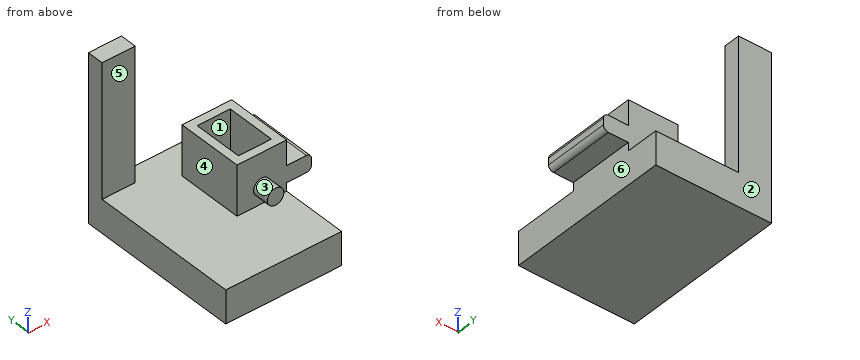
from build123d import *

# Parameters (mm, degrees)
F0_W      = 70
F0_H      = 100
F1_DEPTH  = 20
F2_W      = 20
F2_H      = 10
F3_DEPTH  = 80
F4_W      = 30
F4_H      = 40
F5_DEPTH  = 30
F6_W      = 20
F6_H      = 30
F7_DEPTH  = 30
F8_W      = 40
F8_H      = 10
F9_DEPTH  = 15
F10_R     = 5
F11_DEPTH = 10
F12_R     = 3


with BuildPart() as f1:
    # F0 (on Top) → F1 (new body)
    with BuildSketch(Plane.XY):
        with Locations((35, 50)):
            Rectangle(F0_W, F0_H)
    extrude(amount=F1_DEPTH)

    # F2 (on face) → F3 (join)
    with BuildSketch(Plane.XY.offset(20)):
        with Locations((10, 95)):
            Rectangle(F2_W, F2_H)
    extrude(amount=F3_DEPTH)

    # F4 (on face) → F5 (join)
    with BuildSketch(Plane.XY.offset(20)):
        with Locations((55, 60)):
            Rectangle(F4_W, F4_H)
    extrude(amount=F5_DEPTH)

    # F6 (on face) → F7 (cut)
    with BuildSketch(Plane.XY.offset(50)):
        with Locations((55, 60)):
            Rectangle(F6_W, F6_H)
    extrude(amount=-F7_DEPTH, mode=Mode.SUBTRACT)

    # F8 (on face) → F9 (join)
    with BuildSketch(Plane.YZ.offset(70)):
        with Locations((60, 30)):
            Rectangle(F8_W, F8_H)
    extrude(amount=F9_DEPTH)

    # F10 (on face) → F11 (join)
    with BuildSketch(Plane.XZ.offset(-40)):
        with Locations((55, 30)):
            Circle(F10_R)
    extrude(amount=F11_DEPTH)

    # F12
    f12_edges = [f1.edges().sort_by_distance(p)[0] for p in [
        (85, 60, 35),
        (85, 60, 25),
    ]]
    fillet(f12_edges, radius=F12_R)


solid = f1.part
The listing builds one solid part. Answer for the finished solid, in the listing's coordinates (mm). Face numbers are marked on the shaded views. A direction names the side the tool comes from. Give positions to 0.01 mm unless a question says otherwise; leave off trailing zeros. Loops run counter-clockwise (first coordinate to the right, second up) from the corner with the lowest first, then second, coordinate; pieces in that order, holes last. Notation, with made-up numbers: M 74,-19 L 92,-19 A15 cw 92,3 Z; hole C 0.25,60 d1. An arc over 180 degrees is marked long. Answer as CSV lines item,"result".
Item 1: Given pin 1 Ø10 at (x, y) = (55.5, 61) entering from +Z; pin 2 Ø16 at (x, z) = (54.5, 41.5) entering from +Y; pin 3 Ø10 at (x, y) = (35.5, 32) entering from -Z; pin 4 Ø24 at (x, y) = (62.5, 62) entering from +Z, each flat-ended and moving along its own axis, determine where each tip first touches the part or whether it passes through.
Values follow:
pin 1,"stops at z = 20"
pin 2,"stops at y = 80"
pin 3,"stops at z = 0"
pin 4,"stops at z = 50"
Item 2: Straight lines are drawn through the part: line 1 along Y through (x, z) = (60, 23); line 2 along Y through (x, z) = (59, 32); line 3 along Z through (x, y) = (71.5, 70). For each, find the intervals that lie inside material, in ascending order. Write a range as [from, to].
Values follow:
line 1,"y = [40, 45], [75, 80]"
line 2,"y = [30, 45], [75, 80]"
line 3,"z = [25, 35]"
Item 3: The part is cut by section C-C (y = 61). Give the vertices of the cut face in (x, z), and give its area (3 significant figures).
Values follow:
outline,"M 0,0 L 70,0 L 70,25 L 82,25 A3 ccw 85,28 L 85,32 A3 ccw 82,35 L 70,35 L 70,50 L 65,50 L 65,20 L 45,20 L 45,50 L 40,50 L 40,20 L 0,20 Z"
area,"1,850 mm^2"
Item 4: The mould has two halves that part along X. Classify the marked faces 1, 2 and 3: released by +X, released by -X, zero draft, split by the parting line, or undercut.
Values follow:
face 1,"undercut"
face 2,"zero draft"
face 3,"split by the parting line"
Item 5: The part is cut by section A-A (z = 46.5). Give the vertices of the cut face in (x, y).
Values follow:
outline,"M 0,90 L 20,90 L 20,100 L 0,100 Z; M 40,40 L 70,40 L 70,80 L 40,80 Z; hole M 45,45 L 65,45 L 65,75 L 45,75 Z"
Item 6: The part is cut by section D-D (z = 30). Give the vertices of the cut face in (x, y), and give its area (3 significant figures).
Values follow:
outline,"M 0,90 L 20,90 L 20,100 L 0,100 Z; M 40,40 L 50,40 L 50,30 L 60,30 L 60,40 L 85,40 L 85,80 L 40,80 Z; hole M 45,45 L 65,45 L 65,75 L 45,75 Z"
area,"1,500 mm^2"
Item 7: The part is cut by section B-B (x = 48). Give the vertices of the cut face in (y, z).
Values follow:
outline,"M 0,0 L 100,0 L 100,20 L 80,20 L 80,50 L 75,50 L 75,20 L 45,20 L 45,50 L 40,50 L 40,20 L 0,20 Z"
Item 8: Which of the six approach directions +Z, -Z, +X, -X, +Y, -Y give full straight-line access (tool end or side, diameter ignored) to the marked faces 4, 5 and 6?
Values follow:
face 4,"+Z, -X, +Y, -Y"
face 5,"+Z, +X, -X, -Y"
face 6,"-Z, +X, +Y, -Y"
